from build123d import *

# Parameters (mm, degrees)
SKETCH1_R               = 4
SKETCH1_R_2             = 3.025
BOSS_EXTRUDE1_DEPTH     = 60
SKETCH1_3_R             = 3.025
CUT_EXTRUDE1_DEPTH      = 2.5
CUT_EXTRUDE2_START      = 60
SKETCH1_4_R             = 3.025
CUT_EXTRUDE2_DEPTH      = 2.5
CHAMFER1_SIZE           = 0.25
SKETCH2_R               = 0.875
CUT_EXTRUDE3_DEPTH      = 61.266076693
CUT_EXTRUDE3_DEPTH_BACK = 61.266076693


with BuildPart() as part:
    # Sketch1 → Boss-Extrude1 (new body)
    with BuildSketch(Plane.XY):
        Circle(SKETCH1_R)
        Circle(SKETCH1_R_2, mode=Mode.SUBTRACT)
        Circle(SKETCH1_R_2)
    extrude(amount=BOSS_EXTRUDE1_DEPTH)

    # Sketch1<3> → Cut-Extrude1 (cut)
    with BuildSketch(Plane.XY):
        Circle(SKETCH1_3_R)
    extrude(amount=CUT_EXTRUDE1_DEPTH, mode=Mode.SUBTRACT)

    # Sketch1<4> → Cut-Extrude2 (cut)
    with BuildSketch(Plane.XY.offset(CUT_EXTRUDE2_START)):
        Circle(SKETCH1_4_R)
    extrude(amount=-CUT_EXTRUDE2_DEPTH, mode=Mode.SUBTRACT)

    # Chamfer1
    chamfer1_edges = [part.edges().sort_by_distance(p)[0] for p in [
        (-3.025, 0, 0),
        (-3.025, 0, 60),
    ]]
    chamfer(chamfer1_edges, length=CHAMFER1_SIZE)

    # Sketch2 → Cut-Extrude3 (cut, two sides)
    with BuildSketch(Plane(origin=(0, 0, 0), x_dir=(1, 0, 0), z_dir=(0, 1, 0))) as cut_extrude3_sk:
        with Locations(Location((0, -30, 0), (0, 0, 270))):
            Circle(SKETCH2_R)
    extrude(amount=CUT_EXTRUDE3_DEPTH, mode=Mode.SUBTRACT)
    extrude(cut_extrude3_sk.sketch, amount=-CUT_EXTRUDE3_DEPTH_BACK, mode=Mode.SUBTRACT)


solid = part.part
Design review of the part built by this model. Coordinates are the model's own, in mm. A direction names the side the tool comes from. Give positions to 0.01 mm unless a question says otherwise; leave off trailing zeros. Order: outer loops, then holes, each group sorted by start corner. A loop starts at its lowest first (then second) coordinate and runs counter-clockwise, first axis right, second up. Notation, with made-up numbers: (77.25, -8.75) - (131.25, -8.75) arc R22 ccw to (131.25, 21.25) - close; hole circle Ø1 at (0.5, -23.5). An arc over 180 degrees is marked (long way). Write item = value, one per line. Start each with the question number.
Q1. We need section C-C on z = 11.5. State the section outline as (x, y) points.
Q2. We need section B-B on z = 30. State the section outline as (x, y) points (3 decimals).
Q3. We need section A-A on x = 0. State the section outline as (y, z) points (3 decimals), plus the area to 3 significant figures.
Q4. Tool access review of faces 4 (the face through (-2, -3, 60)), 5 (the face through (2.794, -1.159, 1.359)), 6 (the face through (0, 0, 57.5)): name each direction out of +Z, -Z, +X, -X, +Y, -Y from which nothing blocks a thin tool from reaching the whole face with its end or side.
Q5. Mouldability with a two-part tool opening along X and no side actions: class faces 1 (the face through (-2, -3, 0)), 2 (the face through (1.846, -3.549, 29.58)), 3 (the face through (0, 0, 2.5)) as released by +X, released by -X, zero draft, split by the parting line, or undercut.
Q6. Clearance check with flat-ended pins moving along their axes: pin 1 Ø1.1 at (x, z) = (0, 30) entering from -Y; pin 2 Ø4 at (x, z) = (2, 25) entering from -Y; pin 3 Ø4 at (x, z) = (-2.5, 29) entering from +Y. State where each tip first meets the part, or that it passes through.
Q7. To check wall thickness, follow L1, parallel to Z at x = 0, y = 1.5 (3 decimals); L2, parallel to Y at x = 0, z = 2.05 (3 decimals); L3, parallel to X at y = -2.5, z = 30 (1 decimal). State the ranges of each line that lie inside material, in increasing order. Write a range as from..to.
Working result:
q1.outline = circle Ø8 at (0, 0)
q2.outline = (-0.875, -3.903) - (-0.875, 3.903) arc R4 ccw to start; (0.875, -3.903) arc R4 ccw to (0.875, 3.903) - close
q3.outline = (-4, 0) - (-3.275, 0) - (-3.025, 0.25) - (-3.025, 2.5) - (3.025, 2.5) - (3.025, 0.25) - (3.275, 0) - (4, 0) - (4, 29.125) - (-4, 29.125) - close; (-4, 30.875) - (4, 30.875) - (4, 60) - (3.275, 60) - (3.025, 59.75) - (3.025, 57.5) - (-3.025, 57.5) - (-3.025, 59.75) - (-3.275, 60) - (-4, 60) - close
q3.area = 436 mm²
q4.face_4 = +Z, +X, -X, +Y, -Y
q4.face_5 = -Z
q4.face_6 = +Z
q5.face_1 = zero draft
q5.face_2 = split by the parting line
q5.face_3 = undercut
q6.pin_1 = through
q6.pin_2 = -4
q6.pin_3 = 3.97
q7.L1 = 2.5..29.125, 30.875..57.5
q7.L2 = -4..-3.025, 3.025..4
q7.L3 = -3.1..-0.9, 0.9..3.1
